```python
from build123d import *

# Parameters (mm, degrees)
SKETCH022_W      = 3
SKETCH022_H      = 41
PAD009_DEPTH     = 52
SKETCH023_W      = 3
SKETCH023_H      = 19.3
POCKET011_DEPTH  = 9
SHAPEBINDER008_R = 1.115297
POCKET034_DEPTH  = 5
SHAPEBINDER009_R = 1.382536
POCKET035_DEPTH  = 7.001


with BuildPart() as part:
    # Sketch022 (on ShapeBinder) → Pad009 (new body, symmetric)
    with BuildSketch(Plane(origin=(0, 0, 0), x_dir=(-1, 0, 0), z_dir=(0, 1, 0))):
        with Locations((0, 11.5)):
            Rectangle(SKETCH022_W, SKETCH022_H)
    extrude(amount=PAD009_DEPTH, both=True)

    # Sketch023 (on Face5 of Pad009) → Pocket011 (cut)
    with BuildSketch(Plane.XZ.offset(52)):
        with Locations((0, 0.65)):
            Rectangle(SKETCH023_W, SKETCH023_H)
    extrude(amount=-POCKET011_DEPTH, mode=Mode.SUBTRACT)

    # ShapeBinder008 → Pocket034 (cut)
    with BuildSketch(Plane(origin=(-1.5, -32.5, -4), x_dir=(0, 1, 0), z_dir=(-1, 0, 0))):
        Circle(SHAPEBINDER008_R)
    extrude(amount=-POCKET034_DEPTH, mode=Mode.SUBTRACT)

    # ShapeBinder009 → Pocket035 (cut, through all)
    with BuildSketch(Plane(origin=(-5.5, -43.75, 25.203825), x_dir=(0, 1, 0), z_dir=(-1, 0, 0))):
        Circle(SHAPEBINDER009_R)
    extrude(amount=-POCKET035_DEPTH, mode=Mode.SUBTRACT)


solid = part.part
```
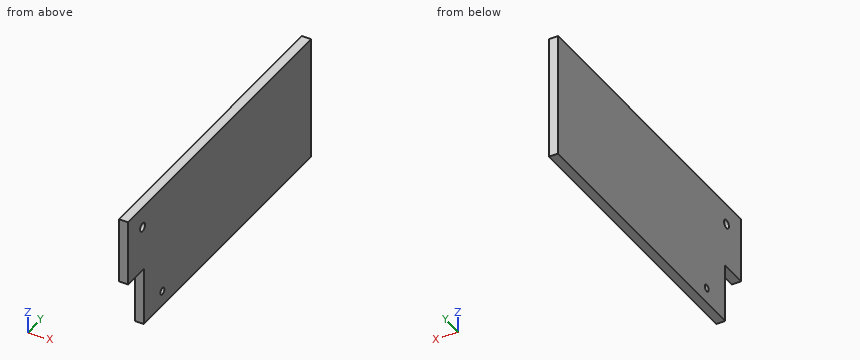
The listing builds one solid part. Answer for the finished solid, in the listing's coordinates (mm). Coordinates: 2 decimals unless noted, no trailing zeros. Write each loop counter-clockwise with the first axis right and the second up, starting at its lowest first coordinate (ties: lowest second). Pieces come first, ordered by that corner, then holes. Notation, with made-up numbers: (11.25, -14.75) - (58.25, -14.75) arc R32 cw to (58.25, 19.25) - close; hole circle Ø11 at (-1, 61.5). An arc over 180 degrees is marked (long way). Return JSON: item names as keys, results as strings. Group by question number.
1. Straight lines are drawn through the part: L1, parallel to Z at x = 0.4, y = -43.75; L2, parallel to Z at x = 0.1, y = -32.5; L3, parallel to Y at x = -0.25, z = -4. For each, find the intervals that lie inside material, in ascending order.
2. A cutting plane is placed at B-B, the plane z = -4. Determine the outline of the cut face in (x, y), plus the area to 3 significant figures.
3. A cutting plane is placed at D-D, the plane z = 0.5. Determine the outline of the cut face in (x, y).
4. A cutting plane is placed at C-C, the plane x = -0.75. Determine the outline of the cut face in (y, z).
5. Given pin 1 (1.5 mm diameter, centred on x = -0.5, y = -47.5, fed in from -Z); pin 2 (2 mm diameter, centred on y = -32.5, z = -4, fed in from +X), each flat-ended and moving along its own axis, determine where each tip first touches the part or whether it passes through.
6. A cutting plane is placed at A-A, the plane y = -32.5. Determine the outline of the cut face in (x, z).
Ans:
{
 "1": {"L1": "10.3 to 23.82, 26.59 to 32", "L2": "-9 to -5.12, -2.88 to 32", "L3": "-43 to -33.62, -31.38 to 52"},
 "2": {"outline": "(-1.5, -43) - (1.5, -43) - (1.5, -33.62) - (-1.5, -33.62) - close; (-1.5, -31.38) - (1.5, -31.38) - (1.5, 52) - (-1.5, 52) - close", "area": "278 mm²"},
 "3": {"outline": "(-1.5, -43) - (1.5, -43) - (1.5, 52) - (-1.5, 52) - close"},
 "4": {"outline": "(-52, 10.3) - (-43, 10.3) - (-43, -9) - (52, -9) - (52, 32) - (-52, 32) - close; hole circle Ø2.77 at (-43.75, 25.2); hole circle Ø2.23 at (-32.5, -4)"},
 "5": {"pin 1": "z = 10.3", "pin 2": "through"},
 "6": {"outline": "(-1.5, -9) - (1.5, -9) - (1.5, -5.12) - (-1.5, -5.12) - close; (-1.5, -2.88) - (1.5, -2.88) - (1.5, 32) - (-1.5, 32) - close"}
}
